Check sheet for the modelled part. Datum: model origin and axes. Units: mm. Face numbers are marked on the shaded views. Round coordinates to 2 decimals unless told otherwise and drop trailing zeros. Loops run counter-clockwise (first coordinate to the right, second up) from the corner with the lowest first, then second, coordinate; pieces in that order, holes last. Notation, with made-up numbers: (40, -21.5) - (89, -21.5) arc R15 cw to (89, -8.5) - close; hole circle Ø1 at (22.5, 86). An arc over 180 degrees is marked (long way). Answer in a Markdown table with one row per item. Add a question column.
(1) Mould release check, pull along Z, two halves, no side actions. Record for the marked faces 1, 2 and 3: +Z half, -Z half, draft (parallel to the pull), parting line (faces both ways), or undercut.
(2) Thickness scan on line 1 along Z through (x, y) = (234.75, -10.5); line 2 along Z through (x, y) = (231.5, -15.5); line 3 along Y through (x, z) = (233, 46.5). Record the ranges inside material, lowest first.
(3) Cross-section at C-C on x = 232.5. Count the separate pieces of the cut face and the enclosed holes in it, then the cut area to 3 significant figures.
(4) Cross-section at A-A on z = 40.5. Enter the section's corners in (x, y).
(5) Cross-section at B-B on z = 55.5. Enter the section's corners in (x, y).
(6) Gauge pin test, flat ends, axial feed: pin 1 (2 mm diameter, centred on y = -21, z = 53, fed in from -X); pin 2 (2 mm diameter, centred on x = 234.5, y = -19, fed in from -Z); pin 3 (3 mm diameter, centred on y = -17, z = 34.5, fed in from +X). Record the tip position at first contact, or that the pin passes through.
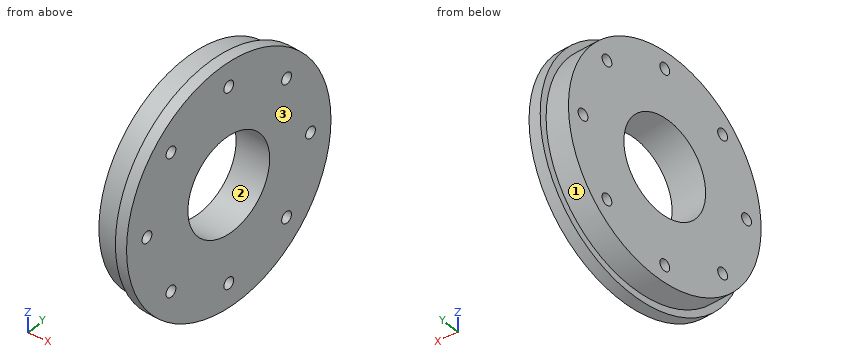
from build123d import *

# Parameters (mm, degrees)
SKETCH1_R           = 14.9606
BOSS_EXTRUDE1_DEPTH = 4.7625
SKETCH2_R           = 6.35
CUT_EXTRUDE1_DEPTH  = 6.35
SKETCH3_R           = 0.762
CUT_EXTRUDE2_DEPTH  = 10
SKETCH5_R           = 15.875
SKETCH5_R_2         = 14.9606
BOSS_EXTRUDE2_DEPTH = 1.5875


with BuildPart() as part:
    # Sketch1 → Boss-Extrude1 (new body)
    with BuildSketch(Plane(origin=(234.278878836, -18.689027227, 0), x_dir=(0, 0, -1), z_dir=(0.9968332748770866, -0.0795199477981641, 0))):
        with Locations(Location((-43.174261814, 8.550344032, 0), (0, 0, 90))):
            Circle(SKETCH1_R)
    extrude(amount=-BOSS_EXTRUDE1_DEPTH)

    # Sketch2 → Cut-Extrude1 (cut)
    with BuildSketch(Plane(origin=(234.278878836, -18.689027227, 0), x_dir=(0, 0, -1), z_dir=(0.9968332748770866, -0.07951994779816411, 0))):
        with Locations(Location((-43.174261814, 8.550344032, 0), (0, 0, 90))):
            Circle(SKETCH2_R)
    extrude(amount=-CUT_EXTRUDE1_DEPTH, mode=Mode.SUBTRACT)

    # Sketch3 → Cut-Extrude2 (cut)
    with BuildSketch(Plane(origin=(229.531460364, -18.310313476, 0), x_dir=(0, 0, 1), z_dir=(-0.9968332748770866, 0.07951994779816411, 0))):
        with Locations(Location((30.474261814, 8.550344032, 0), (0, 0, 270))):
            Circle(SKETCH3_R)
        with Locations(Location((43.174261814, 21.250344032, 0), (0, 0, 270))):
            Circle(SKETCH3_R)
        with Locations(Location((52.154517935, 17.530600153, 0), (0, 0, 270))):
            Circle(SKETCH3_R)
        with Locations(Location((55.874261814, 8.550344032, 0), (0, 0, 270))):
            Circle(SKETCH3_R)
        with Locations(Location((52.154517935, -0.429912089, 0), (0, 0, 270))):
            Circle(SKETCH3_R)
        with Locations(Location((43.174261814, -4.149655968, 0), (0, 0, 270))):
            Circle(SKETCH3_R)
        with Locations(Location((34.194005693, -0.429912089, 0), (0, 0, 270))):
            Circle(SKETCH3_R)
        with Locations(Location((34.194005693, 17.530600153, 0), (0, 0, 270))):
            Circle(SKETCH3_R)
    extrude(amount=-CUT_EXTRUDE2_DEPTH, mode=Mode.SUBTRACT)

    # Sketch5 → Boss-Extrude2 (add)
    with BuildSketch(Plane(origin=(234.278878836, -18.689027227, 0), x_dir=(0, 0, 1), z_dir=(-0.9968332748770866, 0.07951994779816411, 0))):
        with Locations(Location((43.174261814, 8.550344032, 0), (0, 0, 270))):
            Circle(SKETCH5_R)
        with Locations(Location((43.174261814, 8.550344032, 0), (0, 0, 90))):
            Circle(SKETCH5_R_2, mode=Mode.SUBTRACT)
    extrude(amount=BOSS_EXTRUDE2_DEPTH)


solid = part.part
Answers:
| question | item | result |
|---|---|---|
| 1 | face 1 | parting line |
| 1 | face 2 | undercut |
| 1 | face 3 | draft |
| 2 | line 1 | z = 27.3 to 29.8, 31.15 to 36.83, 49.51 to 55.2, 56.55 to 59.05 |
| 2 | line 2 | z = 29.3 to 40.17, 46.18 to 57.05 |
| 2 | line 3 | y = -25.58 to -15.44, -4.58 to 4.62 |
| 3 | separate pieces | 1 |
| 3 | enclosed holes | 9 |
| 3 | area | 586 mm^2 |
| 4 | outline | (229.04, -24.46) - (232.21, -24.71) - (232.13, -25.64) - (233.71, -25.76) - (234.5, -15.91) - (229.75, -15.53) - close; (230.67, -4.05) - (235.42, -4.42) - (236.2, 5.43) - (234.62, 5.56) - (234.55, 4.63) - (231.38, 4.89) - close |
| 5 | outline | (229.54, -18.24) - (232.7, -18.49) - (232.58, -20.01) - (234.16, -20.14) - (234.91, -10.83) - (230.16, -10.45) - close; (230.26, -9.13) - (235.01, -9.5) - (235.75, -0.19) - (234.17, -0.07) - (234.05, -1.59) - (230.89, -1.33) - close |
| 6 | pin 1 | stops at x = 229.27 |
| 6 | pin 2 | stops at z = 29.39 |
| 6 | pin 3 | stops at x = 234.53 |
